```python
from build123d import *

# Parameters (mm, degrees)
SKETCH1_W           = 200
SKETCH1_H           = 100
BOSS_EXTRUDE1_DEPTH = 3
SKETCH2_R           = 1.55
CUT_EXTRUDE1_DEPTH  = 112.843640856
FILLET1_R           = 5
SKETCH3_W           = 10
SKETCH3_H           = 80
SKETCH3_W_2         = 15
SKETCH3_H_2         = 10
CUT_EXTRUDE2_DEPTH  = 112.843640856
FILLET2_R           = 5
FILLET4_R           = 2.5


with BuildPart() as part:
    # Sketch1 → Boss-Extrude1 (new body)
    with BuildSketch(Plane(origin=(0, 0, 0), x_dir=(1, 0, 0), z_dir=(0, 1, 0))):
        Rectangle(SKETCH1_W, SKETCH1_H)
    extrude(amount=BOSS_EXTRUDE1_DEPTH)

    # Sketch2 → Cut-Extrude1 (cut, through all)
    with BuildSketch(Plane(origin=(0, 3, 0), x_dir=(1, 0, 0), z_dir=(0, 1, 0))):
        with Locations(Location((-95, 45, 0), (0, 0, 270))):
            Circle(SKETCH2_R)
        with Locations(Location((-95, -45, 0), (0, 0, 270))):
            Circle(SKETCH2_R)
        with Locations(Location((95, 45, 0), (0, 0, 270))):
            Circle(SKETCH2_R)
        with Locations(Location((95, -45, 0), (0, 0, 270))):
            Circle(SKETCH2_R)
    extrude(amount=-CUT_EXTRUDE1_DEPTH, mode=Mode.SUBTRACT)

    # Fillet1
    fillet1_edges = [part.edges().sort_by_distance(p)[0] for p in [
        (-100, 1.5, -50),
        (100, 1.5, -50),
        (100, 1.5, 50),
        (-100, 1.5, 50),
    ]]
    fillet(fillet1_edges, radius=FILLET1_R)

    # Sketch3 → Cut-Extrude2 (cut, through all)
    with BuildSketch(Plane(origin=(0, 3, 0), x_dir=(1, 0, 0), z_dir=(0, 1, 0))):
        with Locations((95, 0)):
            Rectangle(SKETCH3_W, SKETCH3_H)
        with BuildLine():
            Line((-55.5, 32), (-55.5, 19))
            ThreePointArc((-55.5, 19), (-58, 16.5), (-60.5, 19))
            Line((-60.5, 19), (-60.5, 32))
            ThreePointArc((-60.5, 32), (-58, 34.5), (-55.5, 32))
        make_face()
        with BuildLine():
            Line((-29.365, 26), (-29.365, 16))
            ThreePointArc((-29.365, 16), (-34.365, 11), (-39.365, 16))
            Line((-39.365, 16), (-39.365, 26))
            ThreePointArc((-39.365, 26), (-34.365, 31), (-29.365, 26))
        make_face()
        with Locations((-45.5, 45)):
            Rectangle(SKETCH3_W_2, SKETCH3_H_2)
    extrude(amount=-CUT_EXTRUDE2_DEPTH, mode=Mode.SUBTRACT)

    # Fillet2
    fillet2_edges = [part.edges().sort_by_distance(p)[0] for p in [
        (100, 1.5, 40),
        (100, 1.5, -40),
    ]]
    fillet(fillet2_edges, radius=FILLET2_R - 0.0001)  # a hair under: the kernel refuses the full size

    # Fillet4
    fillet4_edges = [part.edges().sort_by_distance(p)[0] for p in [
        (-38, 1.5, -40),
        (-53, 1.5, -40),
    ]]
    fillet(fillet4_edges, radius=FILLET4_R)


solid = part.part
```
The model under review builds one solid part; all positions refer to its coordinate system, in mm. A direction names the side the tool comes from. Round coordinates to 2 decimals unless told otherwise and drop trailing zeros. Order: outer loops, then holes, each group sorted by start corner. A loop starts at its lowest first (then second) coordinate and runs counter-clockwise, first axis right, second up. Notation, with made-up numbers: (43, 73.5) -> (63, 73.5) arc R25 ccw to (63, 96.5) -> close; hole circle Ø7 at (8.5, 51.5). An arc over 180 degrees is marked (long way). One line per item, written item: value. Start each with the question number.
Q1. Take a section at C-C (z = 34). Write out the cut boundary in (x, y).
Q2. Clearance check with flat-ended pins moving along their axes: pin 1 Ø1.5 at (y, z) = (1, -26) entering from +X; pin 2 Ø0.9 at (y, z) = (2, -47.5) entering from -X. State where each tip first meets the part, or that it passes through.
Q3. Machinability: for faces 1 (the face through (-1, 0, -1)), 2 (the face through (98, 1, 41)), which of the approach directions +Z, -Z, +X, -X, +Y, -Y give a long, thin tool a straight path to every point of the face, cutting with its end or side? Answer none if there is none.
Q4. Wall thickness on line 1 (Z direction, x = 95, y = 0.7); line 2 (X direction, y = 1.9, z = -45); line 3 (Z direction, x = -95, y = 1.75): over which ranges is each line inside the solid? List them lowest first.
Q5. Mouldability with a two-part tool opening along X and no side actions: class faces 3 (the face through (-1, 3, -1)), 4 (the face through (-34.5, 1.5, -31)), 5 (the face through (-99, 2, -48)), 6 (the face through (-34.3, 1.5, -11)) as released by +X, released by -X, zero draft, split by the parting line, or undercut.
Q6. Take a section at B-B (y = 0.75). Count the separate pieces of the cut face and the enclosed holes in it, and give its area (3 significant figures).
Q7. Take a section at A-A (x = -58). Write out the cut boundary in (y, z).
Reported:
1. outline: (-100, 0) -> (90, 0) -> (90, 3) -> (-100, 3) -> close
2. pin 1: stops at x = 90
2. pin 2: stops at x = -99.56
3. face 1: +Z, -Z, +X, -X, -Y
3. face 2: +X, +Y, -Y
4. line 1: z = -50 to -46.55, -43.45 to -40, 40 to 43.45, 46.55 to 50
4. line 2: x = -100 to -96.55, -93.45 to -53, -38 to 93.45, 96.55 to 100
4. line 3: z = -50 to -46.55, -43.45 to 43.45, 46.55 to 50
5. face 3: zero draft
5. face 4: undercut
5. face 5: released by -X
5. face 6: undercut
6. separate pieces: 1
6. enclosed holes: 6
6. area: 18,700 mm2
7. outline: (0, -50) -> (3, -50) -> (3, -34.5) -> (0, -34.5) -> close; (0, -16.5) -> (3, -16.5) -> (3, 50) -> (0, 50) -> close
